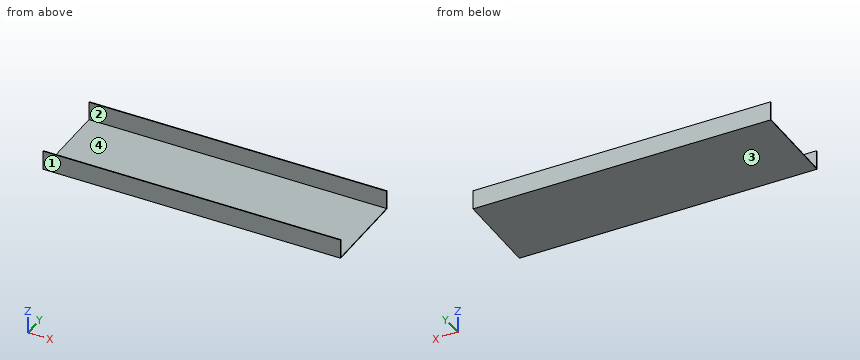
from build123d import *

# Parameters (mm, degrees)
SKETCH_W     = 800
SKETCH_H     = 235
PAD_DEPTH    = 2
SKETCH001_W  = 800
SKETCH001_H  = 2
PAD001_DEPTH = 50


with BuildPart() as part:
    # Sketch → Pad (new body)
    with BuildSketch(Plane.XY):
        Rectangle(SKETCH_W, SKETCH_H)
    extrude(amount=PAD_DEPTH)

    # Sketch001 (on Face6 of Pad) → Pad001 (join)
    with BuildSketch(Plane.XY.offset(2)):
        with Locations((0, 116.5)):
            Rectangle(SKETCH001_W, SKETCH001_H)
        with Locations((0, -116.5)):
            Rectangle(SKETCH001_W, SKETCH001_H)
    extrude(amount=PAD001_DEPTH)


solid = part.part
Work out the finished part from the listing and answer in its coordinate system (mm). Face numbers are marked on the shaded views. Give positions to 0.01 mm unless a question says otherwise; leave off trailing zeros. Order: outer loops, then holes, each group sorted by start corner. A loop starts at its lowest first (then second) coordinate and runs counter-clockwise, first axis right, second up. Notation, with made-up numbers: (88.5, 59) -> (131.5, 59) arc R23 ccw to (131.5, 81) -> close; hole circle Ø4 at (59.25, 26). An arc over 180 degrees is marked (long way). Answer as a JSON object with one key per item and string values. Group by question number.
1. A flat-ended cylindrical pin translates along its axis: pin 1 Ø6 at (x, y) = (-13, -33) entering from +Z. Find the tip coordinate at first contact, or state that the pin passes through.
2. Section C-C on y = 58.5 is taken. Determine the outline of the cut face in (x, z).
3. The mould has two halves that part along Y. Classify the marked faces 1, 2, 3 and 4: released by +Y, released by -Y, zero draft, split by the parting line, or undercut.
4. Consider line 1 along Y through (x, z) = (-149.5, 42); line 2 along Z through (x, y) = (-163, -67.5). Determine where each line is inside the solid, lowest interval first. Write a range as [from, to].
5. Section B-B on x = -191 is taken. Determine the outline of the cut face in (y, z), plus the area to 3 significant figures.
6. Section A-A on z = 23 is taken. Determine the outline of the cut face in (x, y), plus the area to 3 significant figures.
Result sheet:
{
 "1": {"pin 1": "stops at z = 2"},
 "2": {"outline": "(-400, 0) -> (400, 0) -> (400, 2) -> (-400, 2) -> close"},
 "3": {"face 1": "released by -Y", "face 2": "undercut", "face 3": "zero draft", "face 4": "undercut"},
 "4": {"line 1": "y = [-117.5, -115.5], [115.5, 117.5]", "line 2": "z = [0, 2]"},
 "5": {"outline": "(-117.5, 0) -> (117.5, 0) -> (117.5, 52) -> (115.5, 52) -> (115.5, 2) -> (-115.5, 2) -> (-115.5, 52) -> (-117.5, 52) -> close", "area": "670 mm^2"},
 "6": {"outline": "(-400, -117.5) -> (400, -117.5) -> (400, -115.5) -> (-400, -115.5) -> close; (-400, 115.5) -> (400, 115.5) -> (400, 117.5) -> (-400, 117.5) -> close", "area": "3,200 mm^2"}
}
